Geometry check sheet. Reference: the model listing, model coordinates, mm. A direction names the side the tool comes from. Give positions to 0.01 mm unless a question says otherwise; leave off trailing zeros. Loops run counter-clockwise (first coordinate to the right, second up) from the corner with the lowest first, then second, coordinate; pieces in that order, holes last. Notation, with made-up numbers: (9.5, 27) - (36.5, 27) arc R23 cw to (36.5, 38) - close; hole circle Ø5 at (-13, 2.25). An arc over 180 degrees is marked (long way). Use a Markdown table: item, result. Add a question column.
1. Material ranges on L1, parallel to X at y = 39.32, z = 19.45; L2, parallel to X at y = 39.32, z = 6.75; L3, parallel to Y at x = 14, z = 5.25, recorded low to high.
2. Cross-section at C-C on y = -39.32. Enter the section's corners in (x, z), and give its area (3 significant figures).
3. Cross-section at A-A on z = 13.75. Count the separate pieces of the cut face and the enclosed holes in it, and give its area (3 significant figures).
4. Cross-section at D-D on y = -7. Enter the section's corners in (x, z), and give its area (3 significant figures).
5. Set-up check for faces 5 (the flat face through (-38.5, -1, 9)), 6 (the flat face through (-34, -39, 0)): record each of +Z, -Z, +X, -X, +Y, -Y from which the full face is reachable in a straight line by a thin tool's end or side.
6. Depth check by flat-ended pin: P1, Ø2, axis at x = 39.5, z = 13.5, coming from the +Y side; P2, Ø1.5, axis at x = 5.5, y = 7, coming from the -Z side; P3, Ø4, axis at x = 29.5, y = 63, coming from the -Z side. Enter the tip coordinate at first touch or a pass-through.
7. Draft check along Y on faces 1 (the flat face through (0, -74.22, 10)), 2 (the cylindrical face through (-33.4, 40.3, 9.4)), 3 (the flat face through (0, 74.22, 10)), 4 (the cylindrical face through (-33.39, -38.36, 9.43)). Enter one of: pulls with the +Y half, pulls with the -Y half, needs draft (parallel to the pull), parting line crosses it, or undercut.
from build123d import *

# Parameters (mm, degrees)
SKIZZE2_W                       = 148.44
SKIZZE2_H                       = 81
AUFSATZ_LINEAR_AUSTRAGEN1_DEPTH = 20.6
VERRUNDUNG2_R                   = 6
WANDUNG2_T                      = -2
VERST_RKUNGSRIPPE11_START       = -18.6
VERST_RKUNGSRIPPE11_OUTLINE_R   = 2.5
VERST_RKUNGSRIPPE11_OUTLINE_R_2 = 1.5
VERST_RKUNGSRIPPE11_DEPTH       = 18.6
VERST_RKUNGSRIPPE17_START       = -3
VERST_RKUNGSRIPPE17_OUTLINE_R   = 7.6
VERST_RKUNGSRIPPE17_OUTLINE_R_2 = 6.6
VERST_RKUNGSRIPPE17_DEPTH       = 3
SKIZZE31_R                      = 2.698446287
SCHNITT_LINEAR_AUSTRAGEN4_DEPTH = 87.572619228
SKIZZE32_R                      = 1.5
SCHNITT_LINEAR_AUSTRAGEN5_DEPTH = 87.572619228
SKIZZE33_W                      = 25.444588161
SKIZZE33_H                      = 6.979087038
SCHNITT_LINEAR_AUSTRAGEN6_DEPTH = 7


# Read off the part's stored shape, not the designer's step: Verstärkungsrippe11, Verstärkungsrippe17
with BuildPart() as part:
    # Skizze2 → Aufsatz-Linear austragen1 (new body)
    with BuildSketch(Plane(origin=(0, 0, 0), x_dir=(0, 1, 0), z_dir=(0, 0, 1))):
        Rectangle(SKIZZE2_W, SKIZZE2_H)
    extrude(amount=AUFSATZ_LINEAR_AUSTRAGEN1_DEPTH)

    # Verrundung2
    verrundung2_edges = [part.edges().sort_by_distance(p)[0] for p in [
        (40.5, 74.22, 10.3),
        (40.5, -74.22, 10.3),
        (-40.5, -74.22, 10.3),
        (-40.5, 74.22, 10.3),
    ]]
    fillet(verrundung2_edges, radius=VERRUNDUNG2_R)

    # Wandung2
    wandung2_openings = [part.faces().sort_by_distance(p)[0] for p in [
        (0, 0, 0),
    ]]
    offset(amount=WANDUNG2_T, openings=wandung2_openings, kind=Kind.INTERSECTION)

    # Verstärkungsrippe11 outline → Verstärkungsrippe11 (add)
    # profile 1 of 4: a face of its own
    with BuildSketch(Plane(origin=(0, 0, 0), x_dir=(1, 0, 0), z_dir=(0, 0, -1)).offset(VERST_RKUNGSRIPPE11_START)):
        with Locations((-35.7, 39.32)):
            Circle(VERST_RKUNGSRIPPE11_OUTLINE_R)
        with Locations((-35.7, 39.32)):
            Circle(VERST_RKUNGSRIPPE11_OUTLINE_R_2, mode=Mode.SUBTRACT)
    # profile 2 of 4: a face of its own
    with BuildSketch(Plane(origin=(0, 0, 0), x_dir=(1, 0, 0), z_dir=(0, 0, -1)).offset(VERST_RKUNGSRIPPE11_START)):
        with Locations((35.7, 39.32)):
            Circle(VERST_RKUNGSRIPPE11_OUTLINE_R)
        with Locations((35.7, 39.32)):
            Circle(VERST_RKUNGSRIPPE11_OUTLINE_R_2, mode=Mode.SUBTRACT)
    # profile 3 of 4: a face of its own
    with BuildSketch(Plane(origin=(0, 0, 0), x_dir=(1, 0, 0), z_dir=(0, 0, -1)).offset(VERST_RKUNGSRIPPE11_START)):
        with Locations((35.7, -39.32)):
            Circle(VERST_RKUNGSRIPPE11_OUTLINE_R)
        with Locations((35.7, -39.32)):
            Circle(VERST_RKUNGSRIPPE11_OUTLINE_R_2, mode=Mode.SUBTRACT)
    # profile 4 of 4: a face of its own
    with BuildSketch(Plane(origin=(0, 0, 0), x_dir=(1, 0, 0), z_dir=(0, 0, -1)).offset(VERST_RKUNGSRIPPE11_START)):
        with Locations((-35.7, -39.32)):
            Circle(VERST_RKUNGSRIPPE11_OUTLINE_R)
        with Locations((-35.7, -39.32)):
            Circle(VERST_RKUNGSRIPPE11_OUTLINE_R_2, mode=Mode.SUBTRACT)
    extrude(amount=VERST_RKUNGSRIPPE11_DEPTH)

    # Verstärkungsrippe17 outline → Verstärkungsrippe17 (add)
    with BuildSketch(Plane.YX.offset(-15.6).offset(VERST_RKUNGSRIPPE17_START)):
        with Locations((62.650739245, 29.243709866)):
            Circle(VERST_RKUNGSRIPPE17_OUTLINE_R)
        with Locations((62.650739245, 29.243709866)):
            Circle(VERST_RKUNGSRIPPE17_OUTLINE_R_2, mode=Mode.SUBTRACT)
    extrude(amount=VERST_RKUNGSRIPPE17_DEPTH)

    # Skizze31 → Schnitt-Linear austragen4 (cut, through all)
    with BuildSketch(Plane(origin=(0, 0, 18.6), x_dir=(1, 0, 0), z_dir=(0, 0, -1))):
        with Locations(Location((29.243709866, -62.650739245, 0), (0, 0, 180))):
            Circle(SKIZZE31_R)
    extrude(amount=-SCHNITT_LINEAR_AUSTRAGEN4_DEPTH, mode=Mode.SUBTRACT)

    # Skizze32 → Schnitt-Linear austragen5 (cut, through all)
    with BuildSketch(Plane(origin=(0, 0, 18.6), x_dir=(1, 0, 0), z_dir=(0, 0, -1))):
        with Locations((-35.7, 39.32)):
            Circle(SKIZZE32_R)
        with Locations((35.7, 39.32)):
            Circle(SKIZZE32_R)
        with Locations((35.7, -39.32)):
            Circle(SKIZZE32_R)
        with Locations((-35.7, -39.32)):
            Circle(SKIZZE32_R)
    extrude(amount=-SCHNITT_LINEAR_AUSTRAGEN5_DEPTH, mode=Mode.SUBTRACT)

    # Skizze33 → Schnitt-Linear austragen6 (cut)
    with BuildSketch(Plane.YZ.offset(40.5)):
        with Locations((1.502294081, 15.110456481)):
            Rectangle(SKIZZE33_W, SKIZZE33_H)
    extrude(amount=-SCHNITT_LINEAR_AUSTRAGEN6_DEPTH, mode=Mode.SUBTRACT)


solid = part.part
Values found:
| question | item | result |
|---|---|---|
| 1 | L1 | x = -40.5 to -37.2, -34.2 to 34.2, 37.2 to 40.5 |
| 1 | L2 | x = -40.5 to -38.5, -38.2 to -37.2, -34.2 to -33.2, 33.2 to 34.2, 37.2 to 38.2, 38.5 to 40.5 |
| 1 | L3 | y = -74.22 to -72.22, 72.22 to 74.22 |
| 2 | outline | (-40.5, 0) - (-38.5, 0) - (-38.5, 18.6) - (-38.2, 18.6) - (-38.2, 0) - (-37.2, 0) - (-37.2, 20.6) - (-40.5, 20.6) - close; (-34.2, 0) - (-33.2, 0) - (-33.2, 18.6) - (33.2, 18.6) - (33.2, 0) - (34.2, 0) - (34.2, 20.6) - (-34.2, 20.6) - close; (37.2, 0) - (38.2, 0) - (38.2, 18.6) - (38.5, 18.6) - (38.5, 0) - (40.5, 0) - (40.5, 20.6) - (37.2, 20.6) - close |
| 2 | area | 299 mm2 |
| 3 | separate pieces | 5 |
| 3 | enclosed holes | 4 |
| 3 | area | 884 mm2 |
| 4 | outline | (-40.5, 0) - (-38.5, 0) - (-38.5, 18.6) - (40.5, 18.6) - (40.5, 20.6) - (-40.5, 20.6) - close; (38.5, 0) - (40.5, 0) - (40.5, 11.62) - (38.5, 11.62) - close |
| 4 | area | 222 mm2 |
| 5 | face 5 | -Z |
| 5 | face 6 | -Z, +X, -X, +Y, -Y |
| 6 | P1 | stops at y = 72.69 |
| 6 | P2 | stops at z = 18.6 |
| 6 | P3 | passes through |
| 7 | face 1 | pulls with the -Y half |
| 7 | face 2 | undercut |
| 7 | face 3 | pulls with the +Y half |
| 7 | face 4 | undercut |
